Geometry: final body of the model. Coordinates: model frame, mm. A direction names the side the tool comes from. Round coordinates to 2 decimals unless told otherwise and drop trailing zeros. Answer in a Markdown table with one row per item.
```python
from build123d import *

# Parameters (mm, degrees)
ESQUISSE2_R                  = 32.5
BOSS_EXTRU_1_DEPTH           = 25
ESQUISSE3_R                  = 1
ENL_V_MAT_EXTRU_1_DEPTH      = 24
ESQUISSE4_R                  = 26
ENL_V_MAT_EXTRU_2_DEPTH      = 22
ESQUISSE5_R                  = 13
ENL_V_MAT_EXTRU_3_DEPTH      = 51.955863254
ESQUISSE6_R                  = 2
ENL_V_MAT_EXTRU_4_DEPTH      = 51.955863254
BOSS_EXTRU_2_START           = 24
ESQUISSE7_R                  = 1
BOSS_EXTRU_2_DEPTH           = 24
R_P_TITION_CIRCULAIRE1_COUNT = 40
ESQUISSE8_R                  = 2
ENL_V_MAT_EXTRU_5_DEPTH      = 7
R_P_TITION_CIRCULAIRE2_COUNT = 4
ESQUISSE9_R                  = 2
ENL_V_MAT_EXTRU_6_DEPTH      = 7
R_P_TITION_CIRCULAIRE3_COUNT = 4
BOSS_EXTRU_3_START           = -13
ESQUISSE11_R                 = 1.5
BOSS_EXTRU_3_DEPTH           = 13
R_P_TITION_CIRCULAIRE5_COUNT = 4


with BuildPart() as part:
    # Esquisse2 → Boss.-Extru.1 (new body)
    with BuildSketch(Plane.XY):
        Circle(ESQUISSE2_R)
    extrude(amount=BOSS_EXTRU_1_DEPTH)

    # Esquisse3 → Enlèv. mat.-Extru.1 (cut)
    with BuildSketch(Plane.XY.offset(25)):
        with Locations((0, 26)):
            Circle(ESQUISSE3_R)
        with Locations((4.067296091, 25.679896855)):
            Circle(ESQUISSE3_R)
        with Locations((8.034441854, 24.727469424)):
            Circle(ESQUISSE3_R)
        with Locations((11.803752993, 23.166169629)):
            Circle(ESQUISSE3_R)
        with Locations((15.28241656, 21.034441854)):
            Circle(ESQUISSE3_R)
        with Locations((18.384776311, 18.384776311)):
            Circle(ESQUISSE3_R)
        with Locations((21.034441854, 15.28241656)):
            Circle(ESQUISSE3_R)
        with Locations((23.166169629, 11.803752993)):
            Circle(ESQUISSE3_R)
        with Locations((24.727469424, 8.034441854)):
            Circle(ESQUISSE3_R)
        with Locations((25.679896855, 4.067296091)):
            Circle(ESQUISSE3_R)
        with Locations((26, 0)):
            Circle(ESQUISSE3_R)
        with Locations((25.679896855, -4.067296091)):
            Circle(ESQUISSE3_R)
        with Locations((24.727469424, -8.034441854)):
            Circle(ESQUISSE3_R)
        with Locations((23.166169629, -11.803752993)):
            Circle(ESQUISSE3_R)
        with Locations((21.034441854, -15.28241656)):
            Circle(ESQUISSE3_R)
        with Locations((18.384776311, -18.384776311)):
            Circle(ESQUISSE3_R)
        with Locations((15.28241656, -21.034441854)):
            Circle(ESQUISSE3_R)
        with Locations((11.803752993, -23.166169629)):
            Circle(ESQUISSE3_R)
        with Locations((8.034441854, -24.727469424)):
            Circle(ESQUISSE3_R)
        with Locations((4.067296091, -25.679896855)):
            Circle(ESQUISSE3_R)
        with Locations((0, -26)):
            Circle(ESQUISSE3_R)
        with Locations((-4.067296091, -25.679896855)):
            Circle(ESQUISSE3_R)
        with Locations((-8.034441854, -24.727469424)):
            Circle(ESQUISSE3_R)
        with Locations((-11.803752993, -23.166169629)):
            Circle(ESQUISSE3_R)
        with Locations((-15.28241656, -21.034441854)):
            Circle(ESQUISSE3_R)
        with Locations((-18.384776311, -18.384776311)):
            Circle(ESQUISSE3_R)
        with Locations((-21.034441854, -15.28241656)):
            Circle(ESQUISSE3_R)
        with Locations((-23.166169629, -11.803752993)):
            Circle(ESQUISSE3_R)
        with Locations((-24.727469424, -8.034441854)):
            Circle(ESQUISSE3_R)
        with Locations((-25.679896855, -4.067296091)):
            Circle(ESQUISSE3_R)
        with Locations((-26, 0)):
            Circle(ESQUISSE3_R)
        with Locations((-25.679896855, 4.067296091)):
            Circle(ESQUISSE3_R)
        with Locations((-24.727469424, 8.034441854)):
            Circle(ESQUISSE3_R)
        with Locations((-23.166169629, 11.803752993)):
            Circle(ESQUISSE3_R)
        with Locations((-21.034441854, 15.28241656)):
            Circle(ESQUISSE3_R)
        with Locations((-18.384776311, 18.384776311)):
            Circle(ESQUISSE3_R)
        with Locations((-15.28241656, 21.034441854)):
            Circle(ESQUISSE3_R)
        with Locations((-11.803752993, 23.166169629)):
            Circle(ESQUISSE3_R)
        with Locations((-8.034441854, 24.727469424)):
            Circle(ESQUISSE3_R)
        with Locations((-4.067296091, 25.679896855)):
            Circle(ESQUISSE3_R)
    extrude(amount=-ENL_V_MAT_EXTRU_1_DEPTH, mode=Mode.SUBTRACT)

    # Esquisse4 → Enlèv. mat.-Extru.2 (cut)
    with BuildSketch(Plane.XY.offset(25)):
        Circle(ESQUISSE4_R)
    extrude(amount=-ENL_V_MAT_EXTRU_2_DEPTH, mode=Mode.SUBTRACT)

    # Esquisse5 → Enlèv. mat.-Extru.3 (cut, through all)
    with BuildSketch(Plane.XY.offset(3)):
        Circle(ESQUISSE5_R)
    extrude(amount=-ENL_V_MAT_EXTRU_3_DEPTH, mode=Mode.SUBTRACT)

    # Esquisse6 → Enlèv. mat.-Extru.4 (cut, through all)
    with BuildSketch(Plane.XY.offset(3)):
        with Locations((-15.5, 15.5)):
            Circle(ESQUISSE6_R)
        with Locations((15.5, 15.5)):
            Circle(ESQUISSE6_R)
        with Locations((15.5, -15.5)):
            Circle(ESQUISSE6_R)
        with Locations((-15.5, -15.5)):
            Circle(ESQUISSE6_R)
    extrude(amount=-ENL_V_MAT_EXTRU_4_DEPTH, mode=Mode.SUBTRACT)

    # Esquisse7 → Boss.-Extru.2 (add)
    with BuildSketch(Plane.XY.offset(1).offset(BOSS_EXTRU_2_START)):
        with Locations((-21.034441854, 15.28241656)):
            Circle(ESQUISSE7_R)
    boss_extru_2 = extrude(amount=-BOSS_EXTRU_2_DEPTH)

    # Répétition circulaire1: Boss.-Extru.2 ×40 about axis
    r_p_tition_circulaire1_axis = Axis((0, 0, 0), (0, 0, 1))
    for i in range(1, R_P_TITION_CIRCULAIRE1_COUNT):
        add(boss_extru_2.rotate(r_p_tition_circulaire1_axis, i * 360 / R_P_TITION_CIRCULAIRE1_COUNT))

    # Esquisse8 → Enlèv. mat.-Extru.5 (cut)
    with BuildSketch(Plane.XY.offset(25)):
        with Locations((0, 29.25)):
            Circle(ESQUISSE8_R)
    enl_v_mat_extru_5 = extrude(amount=-ENL_V_MAT_EXTRU_5_DEPTH, mode=Mode.SUBTRACT)

    # Répétition circulaire2: Enlèv. mat.-Extru.5 ×4 about axis
    r_p_tition_circulaire2_axis = Axis((0, 0, 0), (0, 0, 1))
    for i in range(1, R_P_TITION_CIRCULAIRE2_COUNT):
        add(enl_v_mat_extru_5.rotate(r_p_tition_circulaire2_axis, i * 360 / R_P_TITION_CIRCULAIRE2_COUNT), mode=Mode.SUBTRACT)

    # Esquisse9 → Enlèv. mat.-Extru.6 (cut)
    with BuildSketch(Plane(origin=(0, 0, 0), x_dir=(-1, 0, 0), z_dir=(0, 0, -1))):
        with Locations((0, 28)):
            Circle(ESQUISSE9_R)
    enl_v_mat_extru_6 = extrude(amount=-ENL_V_MAT_EXTRU_6_DEPTH, mode=Mode.SUBTRACT)

    # Répétition circulaire3: Enlèv. mat.-Extru.6 ×4 about axis
    r_p_tition_circulaire3_axis = Axis((0, 0, 0), (0, 0, 1))
    for i in range(1, R_P_TITION_CIRCULAIRE3_COUNT):
        add(enl_v_mat_extru_6.rotate(r_p_tition_circulaire3_axis, i * 360 / R_P_TITION_CIRCULAIRE3_COUNT), mode=Mode.SUBTRACT)

    # Esquisse11 → Boss.-Extru.3 (add)
    with BuildSketch(Plane.XY.offset(13).offset(BOSS_EXTRU_3_START)):
        with BuildLine():
            Line((-6.644074322, 31.813617782), (-3.368608698, 38))
            Line((-3.368608698, 38), (2.631391302, 38))
            Line((2.631391302, 38), (6.103411428, 31.921753851))
            ThreePointArc((6.103411428, 31.921753851), (-0.275685407, 32.498830711), (-6.644074322, 31.813617782))
        make_face()
        with Locations((-0.368608698, 34.998058912)):
            Circle(ESQUISSE11_R, mode=Mode.SUBTRACT)
    boss_extru_3 = extrude(amount=BOSS_EXTRU_3_DEPTH)

    # Répétition circulaire5: Boss.-Extru.3 ×4 about axis
    r_p_tition_circulaire5_axis = Axis((0, 0, 0), (0, 0, 1))
    for i in range(1, R_P_TITION_CIRCULAIRE5_COUNT):
        add(boss_extru_3.rotate(r_p_tition_circulaire5_axis, i * 360 / R_P_TITION_CIRCULAIRE5_COUNT))


solid = part.part
```
Item 1: First-contact query: P1, Ø6.5, axis at x = 0, y = 28, coming from the -Z side; P2, Ø5, axis at y = -13, z = 19.5, coming from the +X side; P3, Ø1.5, axis at x = 26.5, z = 19, coming from the +Y side; P4, Ø2, axis at x = 0, y = -30, coming from the +Z side. Flat tips, straight axial feed; report the tip coordinate or a pass-through.
Ans:
| item | result |
|---|---|
| P1 | z = 0 |
| P2 | x = 30.76 |
| P3 | y = 19.83 |
| P4 | z = 18 |
Item 2: Mould query, pull axis Y, two halves, no side actions, for faces 3 (the flat face through (34.86, 5.03, 6.41)), 4 (the flat face through (-23, 11, 25)), 5 (the cylindrical face through (3.93, -24.69, 14.15)), 6 (the flat face through (35.003, -4.343, 6.409)). Classes: released by +Y, released by -Y, zero draft, split by the parting line, or undercut.
Ans:
| item | result |
|---|---|
| face 3 | released by +Y |
| face 4 | zero draft |
| face 5 | undercut |
| face 6 | released by -Y |
Item 3: Set-up query: faces 1 (the cylindrical face through (-15.76, -13.517, 1.521)), 2 (the flat face through (29, 0, 18)). Return all of +Z, -Z, +X, -X, +Y, -Y with unobstructed straight access to the full face (end or side cutting, diameter ignored); none if empty.
Ans:
| item | result |
|---|---|
| face 1 | +Z, -Z |
| face 2 | +Z |
Item 4: Ray query, L1, parallel to Y at x = 15.5, z = 2.15; L2, parallel to Z at x = -18, y = -12.5; L3, parallel to Y at x = 11, z = 9.75. Return the intervals inside material, ascending.
Ans:
| item | result |
|---|---|
| L1 | -28.57 to -17.5, -13.5 to 13.5, 17.5 to 28.57 |
| L2 | 0 to 3 |
| L3 | -30.58 to -22.57, 22.57 to 30.58 |
Item 5: Section query A-A, the plane z = 12. State how many separate pieces and enclosed holes the cut face has, and give its area (3 significant figures).
Ans:
| item | result |
|---|---|
| separate pieces | 1 |
| enclosed holes | 5 |
| area | 1,440 mm2 |
